```python
from build123d import *

# Parameters (mm, degrees)
ESQUISSE2_R             = 1.5
ENL_V_MAT_EXTRU_1_DEPTH = 7
ENL_V_MAT_EXTRU_2_REACH = 29
ESQUISSE3_R             = 1.5


with BuildPart() as part:
    # Esquisse1 → Révolution1 (revolve)
    with BuildSketch(Plane.XY):
        Polygon((0, 4.1), (-18, 4.1), (-18, 18), (-12, 18), (-12, 9), (-3, 9), (-3, 7.5), (0, 7.5), align=None)
    revolve(axis=Axis((0, 0, 0), (-1, 0, 0)))

    # Esquisse2 → Enlèv. mat.-Extru.1 (cut, through all)
    with BuildSketch(Plane(origin=(-12, 0, 0), x_dir=(0, 0, -1), z_dir=(1, 0, 0))):
        with Locations((0, 13)):
            Circle(ESQUISSE2_R)
        with Locations((11.258330249, -6.5)):
            Circle(ESQUISSE2_R)
        with Locations((-11.258330249, -6.5)):
            Circle(ESQUISSE2_R)
    extrude(amount=-ENL_V_MAT_EXTRU_1_DEPTH, mode=Mode.SUBTRACT)

    # Esquisse3 → Enlèv. mat.-Extru.2 (cut, up to next)
    with BuildSketch(Plane(origin=(0, 9, 0), x_dir=(1, 0, 0), z_dir=(0, 1, 0)), mode=Mode.PRIVATE) as enl_v_mat_extru_2_sk1:
        with Locations((-7.5, 0)):
            Circle(ESQUISSE3_R)
    enl_v_mat_extru_2_tool1 = extrude(enl_v_mat_extru_2_sk1.sketch, amount=-ENL_V_MAT_EXTRU_2_REACH, mode=Mode.PRIVATE) & part.part
    add(enl_v_mat_extru_2_tool1.solids().sort_by_distance((-7.5, 9, 0))[0], mode=Mode.SUBTRACT)


solid = part.part
```
Geometry check sheet. Reference: the model listing, model coordinates, mm. A direction names the side the tool comes from. Round coordinates to 2 decimals unless told otherwise and drop trailing zeros. Order: outer loops, then holes, each group sorted by start corner. A loop starts at its lowest first (then second) coordinate and runs counter-clockwise, first axis right, second up. Notation, with made-up numbers: M 84.5,15 L 104.5,15 A20 ccw 104.5,29 Z; hole C -39,-4.5 d10. An arc over 180 degrees is marked long. Answer as CSV lines item,"result".
1) Gauge pin test, flat ends, axial feed: pin 1 Ø2.5 at (y, z) = (13, 0) entering from +X; pin 2 Ø3 at (y, z) = (-9, -14) entering from +X; pin 3 Ø3.5 at (y, z) = (-6.5, 11.26) entering from -X; pin 4 Ø10 at (x, z) = (-14, -6) entering from +Y. Record the tip position at first contact, or that the pin passes through.
Entries:
pin 1,"through"
pin 2,"x = -12"
pin 3,"x = -18"
pin 4,"y = 17.97"
2) Tool access check on faces 4 (the face through (-14.958, 11.536, 0.325)), 5 (the face through (-3, -2, -7.4)), 6 (the face through (-9, 6, 0)). Record the directions out of +Z, -Z, +X, -X, +Y, -Y that give a thin tool (end or side, any length) a straight path to the whole face; none if there is none.
Entries:
face 4,"+X, -X"
face 5,"+X"
face 6,"+Y"
3) Sectioned sample at D-D on y = 13. Record the cut outline in (x, z), and give its area (3 significant figures).
Entries:
outline,"M -18,-12.45 L -12,-12.45 L -12,-1.5 L -18,-1.5 Z; M -18,1.5 L -12,1.5 L -12,12.45 L -18,12.45 Z"
area,"131 mm2"
4) Sectioned sample at B-B on z = 0. Record the cut outline in (x, y).
Entries:
outline,"M -18,-18 L -12,-18 L -12,-9 L -3,-9 L -3,-7.5 L 0,-7.5 L 0,-4.1 L -18,-4.1 Z; M -18,4.1 L -9,4.1 L -9,9 L -12,9 L -12,11.5 L -18,11.5 Z; M -18,14.5 L -12,14.5 L -12,18 L -18,18 Z; M -6,4.1 L 0,4.1 L 0,7.5 L -3,7.5 L -3,9 L -6,9 Z"
5) Thickness scan on probe 1 along X at (y, z) = (6.25, 0); probe 2 along X at (y, z) = (-12.5, -9); probe 3 along Y at (x, z) = (-16.5, -1). Record the ranges inside material, lowest first. Write a range as [from, to].
Entries:
probe 1,"[-18, -9], [-6, 0]"
probe 2,"[-18, -12]"
probe 3,"[-17.97, -3.98], [3.98, 11.88], [14.12, 17.97]"
6) Mould release check, pull along Z, two halves, no side actions. Record for faces 1 (the face through (-12, -8.3, -4.3)), 2 (the face through (-14.958, -7.831, 10.566)), 3 (the face through (-7.437, -1.172, -8.923)): +Z half, -Z half, draft (parallel to the pull), parting line (faces both ways), or undercut.
Entries:
face 1,"draft"
face 2,"undercut"
face 3,"parting line"
7) Sectioned sample at C-C on y = -6.5. Record the cut outline in (x, z).
Entries:
outline,"M -18,-16.79 L -12,-16.79 L -12,-12.76 L -18,-12.76 Z; M -18,-9.76 L -12,-9.76 L -12,-6.22 L -3,-6.22 L -3,-3.74 L 0,-3.74 L 0,3.74 L -3,3.74 L -3,6.22 L -12,6.22 L -12,9.76 L -18,9.76 Z; M -18,12.76 L -12,12.76 L -12,16.79 L -18,16.79 Z"
8) Sectioned sample at A-A on y = 0. Record the cut outline in (x, z), and give its area (3 significant figures).
Entries:
outline,"M -18,-18 L -12,-18 L -12,-9 L -3,-9 L -3,-7.5 L 0,-7.5 L 0,-4.1 L -18,-4.1 Z; M -18,4.1 L 0,4.1 L 0,7.5 L -3,7.5 L -3,9 L -12,9 L -12,18 L -18,18 Z"
area,"275 mm2"
